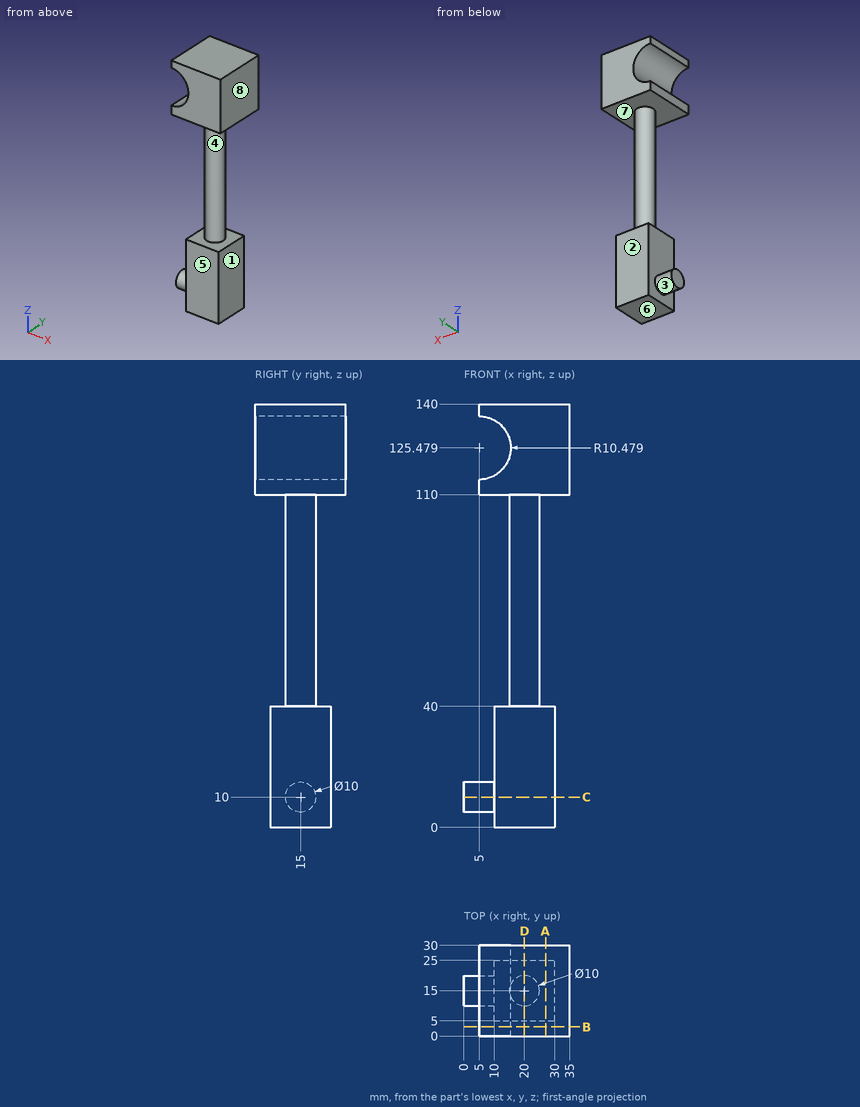
Print and shaded views of the part. All mm, measured from the part's lowest x, y and z. A direction names the side the tool comes from. Coordinates: 2 decimals unless noted, no trailing zeros. Loops run counter-clockwise (first coordinate to the right, second up) from the corner with the lowest first, then second, coordinate; pieces in that order, holes last. Notation, with made-up numbers: (88, -23.75) - (96, -23.75) arc R6 ccw to (96, -19.75) - close; hole circle Ø9 at (64, 11). An arc over 180 degrees is marked (long way). Use one line per item in the form item = value. Start each with the question number.
1) Flat gauge pins, fed straight in: pin 1 (5.5 mm diameter, centred on y = 16.5, z = 113.5, fed in from -X); pin 2 (3 mm diameter, centred on y = 20, z = 60.5, fed in from +X); pin 3 (4 mm diameter, centred on y = 12.5, z = 26, fed in from -X). Where does each tip first touch, or does it go through?
2) Band-saw the part on C-C (z = 10). Give the cut face in (x, y), and give its area (3 significant figures).
3) Drill centre lines: L1, parallel to Z at x = 12.5, y = 20.5; L2, parallel to Z at x = 11, y = 24.25; L3, parallel to Z at x = 20.5, y = 9.25. Where is each one in solid material? Low to high. Write a range as from..to.
4) Tool access for the marked faces 1, 2, 3, 4 and 5: list every direction of +Z, -Z, +X, -X, +Y, -Y with a clear straight run to the whole face (end or side of a thin tool).
5) Band-saw the part on A-A (x = 27). Give the cut face in (y, z), and give its area (3 significant figures).
6) Two-plate mould, pull along Z, no slides. Class the marked faces 6, 7 and 8: +Z half, -Z half, draft (parallel to the pull), parting line (faces both ways), or undercut.
7) Band-saw the part on D-D (x = 20). Give the cut face in (y, z), and give its area (3 significant figures).
8) Band-saw the part on B-B (y = 3). Give the cut face in (x, z).
Check values:
q1.pin_1 = 5
q1.pin_2 = 23.57
q1.pin_3 = 10
q2.outline = (0, 10) - (10, 10) - (10, 5) - (30, 5) - (30, 25) - (10, 25) - (10, 20) - (0, 20) - close
q2.area = 500 mm2
q3.L1 = 0..40, 110..118.16, 132.8..140
q3.L2 = 0..40, 110..116.89, 134.07..140
q3.L3 = 0..40, 110..140
q4.face_1 = -Z, +X, +Y, -Y
q4.face_2 = -Z, +X, -X, +Y
q4.face_3 = -X
q4.face_4 = none
q4.face_5 = -Z, +X, -X, -Y
q5.outline = (0, 110) - (30, 110) - (30, 140) - (0, 140) - close; (5, 0) - (25, 0) - (25, 40) - (5, 40) - close
q5.area = 1,700 mm2
q6.face_6 = -Z half
q6.face_7 = undercut
q6.face_8 = draft
q7.outline = (0, 110) - (10, 110) - (10, 40) - (5, 40) - (5, 0) - (25, 0) - (25, 40) - (20, 40) - (20, 110) - (30, 110) - (30, 140) - (0, 140) - close
q7.area = 2,400 mm2
q8.outline = (5, 110) - (35, 110) - (35, 140) - (5, 140) - (5, 135.96) arc R10.48 cw to (5, 115) - close
